Geometry: see drawing. Coordinates: mm, zero at the bounding-box minimum. A direction names the side the tool comes from. Give positions to 0.01 mm unless a question says otherwise; leave off trailing zeros. Write each loop counter-clockwise with the first axis right and the second up, starting at its lowest first coordinate (ties: lowest second). Pieces come first, ordered by that corner, then holes.
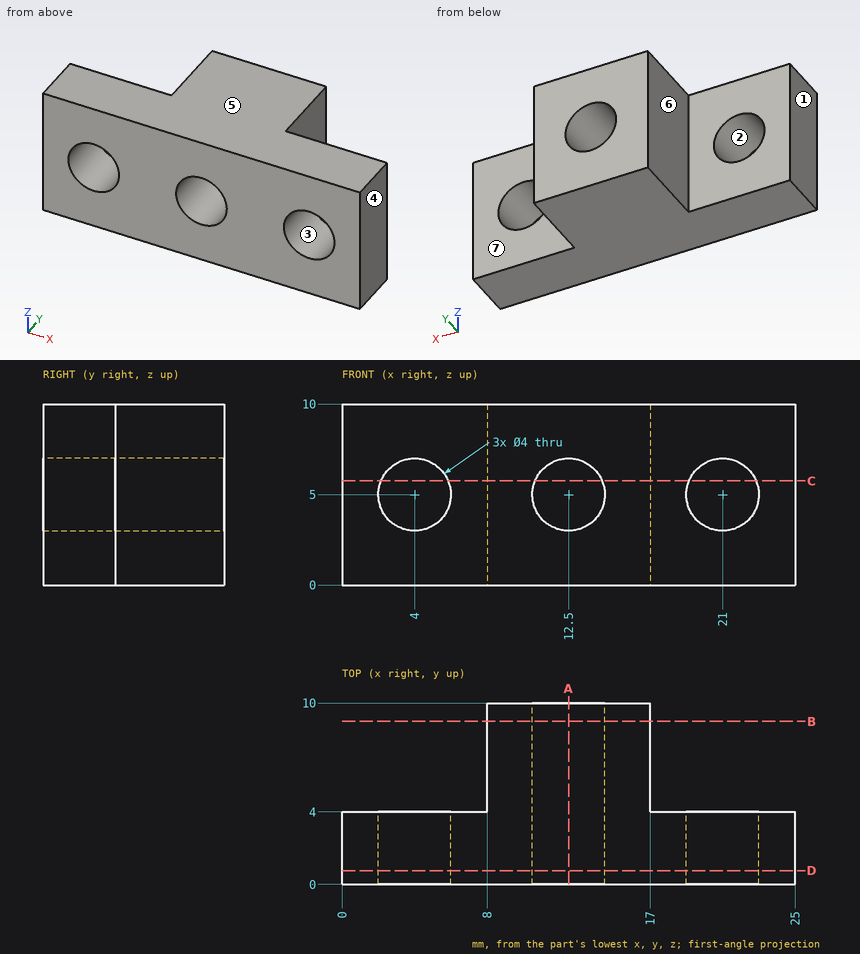
Q1. Section C-C, the plane z = 5.75. Return the cut outline in (x, y), then the cut area to 3 significant figures.
Q2. Material intervals for line 1 along X through (y, z) = (2, 5); line 2 along X through (y, z) = (6.25, 5); line 3 along X through (y, z) = (1.25, 5.5), sorted ascending.
Q3. Section A-A, the plane x = 12.5. Return the cut outline in (y, z).
Q4. Mould query, pull axis X, two halves, no side actions, for the marked faces 1, 2, 3 and 4. Classes: +X half, -X half, draft (parallel to the pull), parting line (faces both ways), or undercut.
Q5. Access query for the marked faces 5, 6 and 7. Directions: +Z, -Z, +X, -X, +Y, -Y. A direction counts if a zero-diameter tool reaches every point of the face in a straight line with its end or side. Return the directions, or none.
Q6. Section B-B, the plane y = 9. Return the cut outline in (x, z).
Q7. Pin query (flat end, axial travel): pin 1 (2.5 mm diameter, centred on x = 2.5, z = 6, fed in from +Y); pin 2 (1.5 mm diameter, centred on y = 6.5, z = 3.5, fed in from +X); pin 3 (2.5 mm diameter, centred on x = 4, z = 5, fed in from +Y); pin 4 (5 mm diameter, centred on y = 8, z = 7.5, fed in from -X). Return the tip coordinate at first contact, or that it passes through.
Q8. Section D-D, the plane y = 0.75. Return the cut outline in (x, z).
Solutions:
1. outline: (0, 0) - (2.15, 0) - (2.15, 4) - (0, 4) - close; (5.85, 0) - (10.65, 0) - (10.65, 10) - (8, 10) - (8, 4) - (5.85, 4) - close; (14.35, 0) - (19.15, 0) - (19.15, 4) - (17, 4) - (17, 10) - (14.35, 10) - close; (22.85, 0) - (25, 0) - (25, 4) - (22.85, 4) - close
1. area: 87.3 mm2
2. line 1: x = 0 to 2, 6 to 10.5, 14.5 to 19, 23 to 25
2. line 2: x = 8 to 10.5, 14.5 to 17
2. line 3: x = 0 to 2.06, 5.94 to 10.56, 14.44 to 19.06, 22.94 to 25
3. outline: (0, 0) - (10, 0) - (10, 3) - (0, 3) - close; (0, 7) - (10, 7) - (10, 10) - (0, 10) - close
4. face 1: -X half
4. face 2: undercut
4. face 3: undercut
4. face 4: +X half
5. face 5: +Z, +X, -X, +Y, -Y
5. face 6: +Z, -Z, -X, +Y
5. face 7: +Z, -Z, +X, +Y
6. outline: (8, 0) - (17, 0) - (17, 10) - (8, 10) - close; hole circle Ø4 at (12.5, 5)
7. pin 1: stops at y = 4
7. pin 2: stops at x = 17
7. pin 3: passes through
7. pin 4: stops at x = 8
8. outline: (0, 0) - (25, 0) - (25, 10) - (0, 10) - close; hole circle Ø4 at (4, 5); hole circle Ø4 at (12.5, 5); hole circle Ø4 at (21, 5)
